Geometry check sheet. Reference: drawing and pictorial views, mm from the part's lowest x, y, z. A direction names the side the tool comes from. Coordinates: 2 decimals unless noted, no trailing zeros. Loops run counter-clockwise (first coordinate to the right, second up) from the corner with the lowest first, then second, coordinate; pieces in that order, holes last. Notation, with made-up numbers: (43, 78.5) -> (72, 78.5) arc R32 ccw to (72, 110.5) -> close; hole circle Ø6 at (-29, -24.5). An arc over 180 degrees is marked (long way). Answer as a JSON object with one key per item and string values. Group by question number.
Q1. Scan lines: L1, parallel to Y at x = 15, z = 2.1; L2, parallel to Z at x = 23.25, y = 13.25; L3, parallel to X at y = 14.5, z = 1.35. Record each from-to range of solid material in increasing order.
Q2. Cross-section at D-D on y = 27. Record the boundary of the cut face in (x, z).
Q3. Release check for a two-part mould opening along Y. For the marked faces 1 and 2 record: released by +Y, released by -Y, zero draft, split by the parting line, or undercut.
Q4. Cross-section at C-C on z = 2.35. Record the boundary of the cut face in (x, y), and give its area (3 significant figures).
Q5. Cross-section at B-B on y = 15. Record the boundary of the cut face in (x, z).
Q6. Cross-section at A-A on x = 15. Record the boundary of the cut face in (y, z).
Q7. Set-up check for the marked faces 3, 4 and 5: record each of +Z, -Z, +X, -X, +Y, -Y from which the full face is reachable in a straight line by a thin tool's end or side.
Q8. Gauge pin test, flat ends, axial feed: pin 1 Ø0.9 at (y, z) = (14, 1) entering from +X; pin 2 Ø12 at (x, y) = (24.5, 5.5) entering from -Z; pin 3 Ø9 at (x, y) = (10, 20.5) entering from -Z. Record the tip position at first contact, or that the pin passes through.
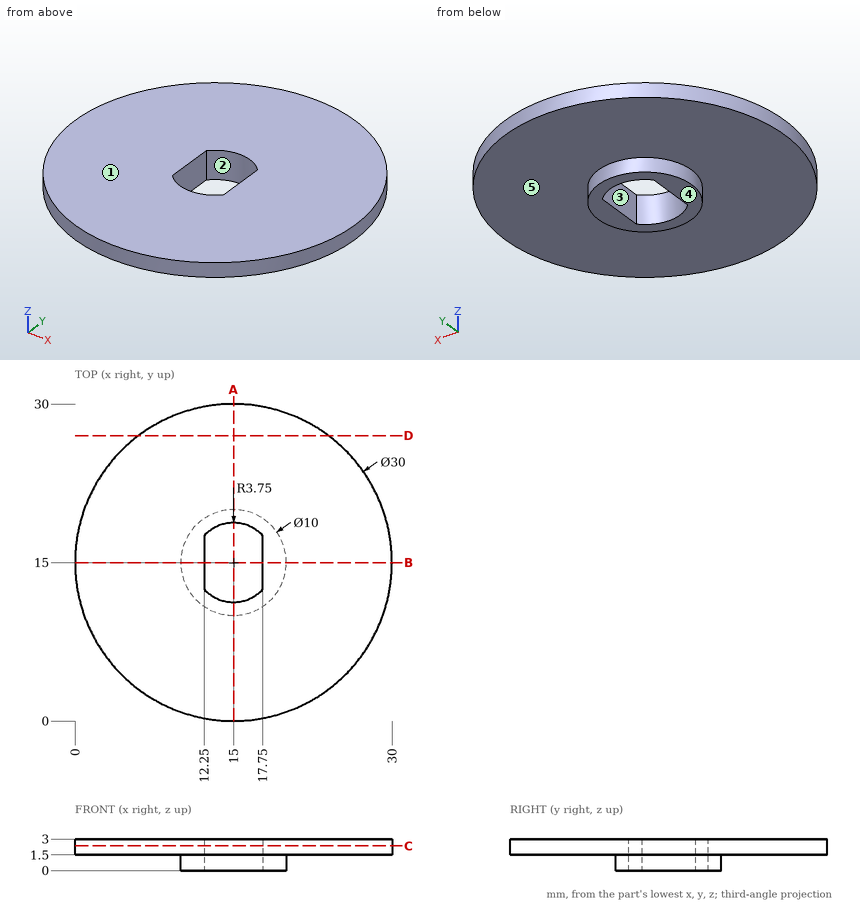
Computed values:
{
 "1": {"L1": "y = 0 to 11.25, 18.75 to 30", "L2": "z = 1.5 to 3", "L3": "x = 10.03 to 12.25, 17.75 to 19.97"},
 "2": {"outline": "(6, 1.5) -> (24, 1.5) -> (24, 3) -> (6, 3) -> close"},
 "3": {"face 1": "zero draft", "face 2": "undercut"},
 "4": {"outline": "circle Ø30 at (15, 15); hole (12.25, 12.45) arc R3.75 ccw to (17.75, 12.45) -> (17.75, 17.55) arc R3.75 ccw to (12.25, 17.55) -> close", "area": "670 mm²"},
 "5": {"outline": "(0, 1.5) -> (10, 1.5) -> (10, 0) -> (12.25, 0) -> (12.25, 3) -> (0, 3) -> close; (17.75, 0) -> (20, 0) -> (20, 1.5) -> (30, 1.5) -> (30, 3) -> (17.75, 3) -> close"},
 "6": {"outline": "(0, 1.5) -> (10, 1.5) -> (10, 0) -> (11.25, 0) -> (11.25, 3) -> (0, 3) -> close; (18.75, 0) -> (20, 0) -> (20, 1.5) -> (30, 1.5) -> (30, 3) -> (18.75, 3) -> close"},
 "7": {"face 3": "+Z, -Z", "face 4": "-Z, +X, -X, +Y, -Y", "face 5": "-Z"},
 "8": {"pin 1": "stops at x = 19.97", "pin 2": "stops at z = 1.5", "pin 3": "stops at z = 0"}
}
